The listing builds one solid part. Answer for the finished solid, in the listing's coordinates (mm). A direction names the side the tool comes from. Round coordinates to 2 decimals unless told otherwise and drop trailing zeros. Write each loop counter-clockwise with the first axis right and the second up, starting at its lowest first coordinate (ties: lowest second). Pieces come first, ordered by that corner, then holes.
(1) A cutting plane is placed at B-B, the plane y = 0.7. Give the vertices of the cut face in (x, z).
(2) A cutting plane is placed at C-C, the plane x = 5.75. Give the vertices of the cut face in (y, z), and give its area (3 significant figures).
(3) Find the intervals of material crossed by probe 1 along Z at (x, y) = (-10.25, 0.2); probe 2 along X at (y, z) = (0.9, 0); probe 3 along Y at (x, z) = (-2.5, 0.75), in increasing order.
(4) Each of these flat-tipped pins is pushed along its axis until it touches: pin 1 Ø1 at (y, z) = (1.5, -1.5) entering from +X; pin 2 Ø1 at (x, y) = (2.5, 1) entering from +Z; pin 3 Ø3 at (x, y) = (-6.5, 0.5) entering from -Z. Where does it stop, or does it pass through?
(5) For faces 4 (the face through (-5, 1, -2.5)), 5 (the face through (0, 1, 2)), 6 (the face through (0, 1, -2)), determine the directions among +Z, -Z, +X, -X, +Y, -Y from which every point of the face is accessible in a straight line to the end or side of a thin tool.
(6) The mould has two halves that part along X. Classify faces 1 (the face through (-9, 1, 0)), 2 (the face through (-5, 1, 2.5)), 3 (the face through (-12.5, 1, 0.1)): +X half, -X half, draft (parallel to the pull), parting line (faces both ways), or undercut.
(7) A cutting plane is placed at D-D, the plane z = -1.7. Give the vertices of the cut face in (x, y), and give its area (3 significant figures).
(8) A cutting plane is placed at A-A, the plane z = 0. Give the vertices of the cut face in (x, y).
from build123d import *

# Parameters (mm, degrees)
SKETCH1_R               = 1
BOSS_EXTRUDE1_DEPTH     = 2
SKETCH4_W               = 2
SKETCH4_H               = 2
BOSS_EXTRUDE2_DEPTH     = 11
CUT_EXTRUDE1_DEPTH      = 13.903487901
CUT_EXTRUDE1_DEPTH_BACK = 13.903487901
CUT_EXTRUDE2_DEPTH      = 14.133925537
CUT_EXTRUDE2_DEPTH_BACK = 14.133925537
CUT_EXTRUDE3_DEPTH      = 14.133925537
CUT_EXTRUDE3_DEPTH_BACK = 14.133925537
SKETCH7_R               = 0.5


with BuildPart() as part:
    # Sketch1 → Boss-Extrude1 (new body)
    with BuildSketch(Plane(origin=(0, 0, 0), x_dir=(1, 0, 0), z_dir=(0, 1, 0))):
        with BuildLine():
            Line((-10, 2.5), (0, 2.5))
            Line((0, 2.5), (0, -2.5))
            Line((0, -2.5), (-10, -2.5))
            ThreePointArc((-10, -2.5), (-12.5, 0), (-10, 2.5))
        make_face()
        with Locations(Location((-10, 0, 0), (0, 0, 270))):
            Circle(SKETCH1_R, mode=Mode.SUBTRACT)
    extrude(amount=BOSS_EXTRUDE1_DEPTH)

    # Sketch4 → Boss-Extrude2 (add)
    with BuildSketch(Plane(origin=(0, 0, 0), x_dir=(0, 0, -1), z_dir=(1, 0, 0))):
        with Locations((0, 1)):
            Rectangle(SKETCH4_W, SKETCH4_H)
    extrude(amount=BOSS_EXTRUDE2_DEPTH)

    # Sketch5 → Cut-Extrude1 (cut, two sides: drawn at the far end of the back side and taken through both)
    with BuildSketch(Plane(origin=(0, 2, 0), x_dir=(1, 0, 0), z_dir=(0, 1, 0)).offset(-CUT_EXTRUDE1_DEPTH_BACK)):
        with BuildLine():
            Line((10, 1), (10, 1.5))
            Line((10, 1.5), (12, 1.5))
            Line((12, 1.5), (12, -1.5))
            Line((12, -1.5), (10, -1.5))
            Line((10, -1.5), (10, -1))
            ThreePointArc((10, -1), (11, 0), (10, 1))
        make_face()
    extrude(amount=CUT_EXTRUDE1_DEPTH + CUT_EXTRUDE1_DEPTH_BACK, mode=Mode.SUBTRACT)

    # Sketch6 → Cut-Extrude2 (cut, two sides: drawn at the far end of the back side and taken through both)
    with BuildSketch(Plane(origin=(0, 0, -1), x_dir=(-1, 0, 0), z_dir=(0, 0, -1)).offset(-CUT_EXTRUDE2_DEPTH_BACK)):
        with BuildLine():
            Line((-10, 2), (-10, 2.5))
            Line((-10, 2.5), (-12, 2.5))
            Line((-12, 2.5), (-12, -0.5))
            Line((-12, -0.5), (-10, -0.5))
            Line((-10, -0.5), (-10, 0))
            ThreePointArc((-10, 0), (-11, 1), (-10, 2))
        make_face()
    extrude(amount=CUT_EXTRUDE2_DEPTH + CUT_EXTRUDE2_DEPTH_BACK, mode=Mode.SUBTRACT)

    # Sketch7 → Cut-Extrude3 (cut, two sides: drawn at the far end of the back side and taken through both)
    with BuildSketch(Plane(origin=(0, 0, -1), x_dir=(-1, 0, 0), z_dir=(0, 0, -1)).offset(-CUT_EXTRUDE3_DEPTH_BACK)):
        with Locations(Location((-10, 1, 0), (0, 0, 90))):
            Circle(SKETCH7_R)
    extrude(amount=CUT_EXTRUDE3_DEPTH + CUT_EXTRUDE3_DEPTH_BACK, mode=Mode.SUBTRACT)

    # Sketch10 → Revolve1 (revolve)
    with BuildSketch(Plane.XY):
        with BuildLine():
            ThreePointArc((10, 3.75), (12.75, 1), (10, -1.75))
            Line((10, -1.75), (10, 1))
            Line((10, 1), (10, 3.75))
        make_face()
    revolve(axis=Axis((10, 1, 0), (0, 1, 0)))


solid = part.part
Solutions:
1. outline: (-10, -2.5) - (0, -2.5) - (0, -1) - (7.46, -1) arc R2.73 ccw (long way) to (7.46, 1) - (0, 1) - (0, 2.5) - (-10, 2.5) arc R2.5 ccw to start; hole circle Ø2 at (-10, 0)
2. outline: (0, -1) - (2, -1) - (2, 1) - (0, 1) - close
2. area: 4.00 mm2
3. probe 1: z = -2.49 to -0.97, 0.97 to 2.49
3. probe 2: x = -12.5 to -11, -9 to 12.75
3. probe 3: y = 0 to 2
4. pin 1: stops at x = 12.53
4. pin 2: stops at z = 1
4. pin 3: stops at z = -2.5
5. face 4: -Z, -X, +Y, -Y
5. face 5: +Z, +Y, -Y
5. face 6: -Z, +Y, -Y
6. face 1: undercut
6. face 2: draft
6. face 3: -X half
7. outline: (-11.83, 0) - (0, 0) - (0, 2) - (-11.83, 2) - close; circle Ø4.32 at (10, 1)
7. area: 38.3 mm2
8. outline: (-12.5, 0) - (-11, 0) - (-11, 2) - (-12.5, 2) - close; (-9, 0) - (7.44, 0) arc R2.75 ccw (long way) to (7.44, 2) - (-9, 2) - close
